Read the model definition and answer for the solid it produces. Units are mm, in the model's axes. A direction names the side the tool comes from. Coordinates: 2 decimals unless noted, no trailing zeros. Write each loop counter-clockwise with the first axis right and the second up, starting at its lowest first coordinate (ties: lowest second). Pieces come first, ordered by that corner, then holes.
(1) Which of the six approach directions +Z, -Z, +X, -X, +Y, -Y give full straight-line access (tool end or side, diameter ignored) to faces 4 (the flat face through (-49, -5.75, 4)), 5 (the cylindrical face through (46.38, 6.13, 5.05)), 6 (the flat face through (-49, 0, 5.4)), 7 (the flat face through (-49, 0, 5.6)), 8 (the flat face through (-17, 19.5, 4))?
(2) The part is cut by section D-D, the plane x = 31.6. Determine the outline of the cut face in (y, z).
(3) The part is cut by section A-A, the plane x = -48.85. Determine the outline of the cut face in (y, z) (3 decimals), and give its area (3 significant figures).
(4) Straight lines are drawn through the part: line 1 along Y through (x, z) = (46.1, 1.05); line 2 along Y through (x, z) = (5, 6); line 3 along Y through (x, z) = (-48.85, 0.85) (3 decimals). For each, find the intervals that lie inside material, in ascending order.
(5) Given pin 1 (4 mm diameter, centred on x = -48, y = 1.5, fed in from +Z); pin 2 (5.5 mm diameter, centred on x = 46.1, y = -19.5, fed in from +Z); pin 3 (0.7 mm diameter, centred on y = 1.5, z = 4.5, fed in from -X); pin 4 (1.5 mm diameter, centred on y = -18.5, z = 2.5, fed in from -X), each flat-ended and moving along its own axis, determine where each tip first touches the part or whether it passes through.
(6) The part is cut by section B-B, the plane y = -19.5. Determine the outline of the cut face in (x, z).
(7) The part is cut by section C-C, the plane y = 0. Determine the outline of the cut face in (x, z).
(8) Determine the mould class of faces 1 (the flat face through (-19, -14, 6.6)), 2 (the flat face through (-49, 0, 4.1)), 3 (the flat face through (-16, -14.5, 4)) for opening direction Y: pulls with the +Y half, pulls with the -Y half, needs draft (parallel to the pull), parting line crosses it, or undercut.
Autodesk Inventor part; units mm, degrees
ref_plane "YZ Plane" through (0, 0, 0) normal (1, 0, 0) x (0, 1, 0)
ref_plane "XZ Plane" through (0, 0, 0) normal (0, 1, 0) x (-1, 0, 0)
ref_plane "XY Plane" through (0, 0, 0) normal (0, 0, 1) x (1, 0, 0)
sketch "Sketch1" plane through (0, 0, 0) normal (0, 0, 1) x (1, 0, 0)
  line L0 (-52.6, 23) -> (52.6, 23)
  line L1 (52.6, 23) -> (52.6, -23)
  line L2 (52.6, -23) -> (-52.6, -23)
  line L3 (-52.6, -23) -> (-52.6, 23)
  point P0 (0, 0)
  point P1 (-52.6, 0)
  point P2 (0, 23)
  dimension "d0" = 105.2
  dimension "d2" = 46
extrude "Extrusion1" add sketch "Sketch1" along normal blind 1.6
sketch "Sketch2" plane through (0, 0, 1.6) normal (0, 0, 1) x (1, 0, 0)
  line L0 (-52.6, -23) -> (52.6, -23)
  line L1 (52.6, -23) -> (52.6, 23)
  line L2 (-45.1, 19.5) -> (12.4, 19.5)
  line L3 (12.4, 19.5) -> (12.4, -14.5)
  line L4 (12.4, -14.5) -> (-45.1, -14.5)
  line L5 (-45.1, -14.5) -> (-45.1, 19.5)
  circle A0 centre (31.6, 0) radius 16
  line L6 (31.6, 0) -> (31.6, -16)
  line L7 (31.6, 0) -> (31.6, 16)
  line L8 (52.6, 23) -> (-52.6, 23)
  line L9 (-52.6, 23) -> (-52.6, -23)
  point P0 (0, 0)
  dimension "d5" = 57.5
  dimension "d7" = 34
  dimension "d8" = 32
  dimension "d9" = 21
  dimension "d10" = 23
  dimension "d13" = 3.5
  dimension "d14" = 7.5
extrude "Extrusion2" add sketch "Sketch2" along normal blind 7 contours L2 L3 L4 L5 | A0 L6 L7 | L7 L6 A0
sketch "Sketch3" plane through (0, 0, 8.6) normal (0, 0, 1) x (1, 0, 0)
  line L0 (12.4, 19.5) -> (-45.1, 19.5)
  line L1 (-45.1, 19.5) -> (-45.1, -14.5)
  line L2 (-45.1, -14.5) -> (12.4, -14.5)
  line L3 (12.4, -14.5) -> (12.4, 19.5)
  point P0 (0, 0)
extrude "Extrusion3" cut sketch "Sketch3" against normal blind 2
sketch "Sketch4" plane through (0, 0, 6.6) normal (0, 0, 1) x (1, 0, 0)
  line L0 (-45.1, 19.5) -> (12.4, 19.5)
  line L1 (-45.1, -14.5) -> (-45.1, 19.5)
  line L2 (-42.5865, 18.0138) -> (9.8865, 18.0138)
  line L3 (9.8865, 18.0138) -> (9.8865, -13.0138)
  line L4 (9.8865, -13.0138) -> (-42.5865, -13.0138)
  line L5 (-42.5865, -13.0138) -> (-42.5865, 18.0138)
  line L6 (-45.1, -14.5) -> (-42.5865, -13.0138) construction
  point P0 (0, 0)
  point P1 (-45.1, 2.5)
  point P2 (-42.5865, 2.5)
  point P3 (-16.35, 18.0138)
  point P4 (-16.35, 19.5)
  dimension "d21" = 60.96
extrude "Extrusion4" cut sketch "Sketch4" against normal blind 1
sketch "Sketch5" plane through (0, 0, 1.6) normal (0, 0, 1) x (1, 0, 0)
  line L0 (-52.6, 23) -> (-52.6, -23)
  line L1 (-52.6, -5.75) -> (-45.1, -5.75)
  line L2 (-45.1, -5.75) -> (-45.1, 5.75)
  line L3 (-45.1, 5.75) -> (-52.6, 5.75)
  line L4 (-52.6, 5.75) -> (-52.6, -5.75)
  line L5 (-45.1, -14.5) -> (-45.1, 19.5)
  point P0 (0, 0)
  point P1 (-45.1, 0)
  point P2 (-52.6, 0)
  dimension "d24" = 11.5
extrude "Extrusion5" add sketch "Sketch5" along normal blind 4
sketch "Sketch6" plane through (-52.6, -23, 0) normal (-1, 0, 0) x (0, 0, 1)
  line L0 (1.6, 17.25) -> (5.6, 17.25)
  line L1 (5.6, 28.75) -> (5.6, 17.25)
  line L2 (1.6, 28.75) -> (5.6, 28.75)
  line L3 (1.6, 46) -> (1.6, 28.75)
  line L4 (4.1, 28.55) -> (5.4, 28.55)
  line L5 (5.4, 28.55) -> (5.4, 17.45)
  line L6 (5.4, 17.45) -> (4.1, 17.45)
  line L7 (4.1, 17.45) -> (4.1, 28.55)
  point P0 (0, 23)
  dimension "d28" = 2.5
  dimension "d29" = 0.2
  dimension "d30" = 0.2
  dimension "d31" = 0.2
extrude "Extrusion6" cut sketch "Sketch6" against normal up to surface (7.5 mm away)
sketch "Sketch7" plane through (0, 0, 1.6) normal (0, 0, 1) x (1, 0, 0)
  line L0 (52.6, -23) -> (52.6, 23)
  line L1 (-52.6, 23) -> (-52.6, 5.75)
  line L2 (-45.1, -14.5) -> (-45.1, -5.75)
  circle A0 centre (-48.85, -10.125) radius 1.75
  circle A1 centre (-48.85, 10.125) radius 1.75
  circle A2 centre (46.1, 19.5) radius 1.75
  circle A3 centre (46.1, -19.5) radius 1.75
  line L3 (-48.85, 10.125) -> (-48.85, -10.125) construction
  line L4 (46.1, 19.5) -> (46.1, -19.5) construction
  point P0 (0, 0)
  point P1 (52.6, 0)
  point P2 (-48.85, 0)
  point P3 (46.1, 0)
  point P4 (52.6, 0)
  point P5 (52.6, 0)
  dimension "d34" = 20.25
  dimension "d36" = 3.75
  dimension "d37" = 39
  dimension "d39" = 6.5
  dimension "d40" = 3.5
extrude "Extrusion7" cut sketch "Sketch7" against normal through all
properties part number "miniviki"
Computed:
1. face 4: +Z, -X, -Y
1. face 5: +Z
1. face 6: -X
1. face 7: +Z, -X, +Y, -Y
1. face 8: +Z, +X, -X, +Y
2. outline: (-23, 0) - (23, 0) - (23, 1.6) - (16, 1.6) - (16, 8.6) - (-16, 8.6) - (-16, 1.6) - (-23, 1.6) - close
3. outline: (-23, 0) - (-11.875, 0) - (-11.875, 1.6) - (-23, 1.6) - close; (-8.375, 0) - (8.375, 0) - (8.375, 1.6) - (5.75, 1.6) - (5.75, 5.6) - (-5.75, 5.6) - (-5.75, 1.6) - (-8.375, 1.6) - close; (11.875, 0) - (23, 0) - (23, 1.6) - (11.875, 1.6) - close; hole (-5.55, 4.1) - (5.55, 4.1) - (5.55, 5.4) - (-5.55, 5.4) - close
3. area: 94.0 mm2
4. line 1: y = -23 to -21.25, -17.75 to 17.75, 21.25 to 23
4. line 2: y = -14.5 to -13.01, 18.01 to 19.5
4. line 3: y = -23 to -11.875, -8.375 to 8.375, 11.875 to 23
5. pin 1: stops at z = 5.6
5. pin 2: stops at z = 1.6
5. pin 3: stops at x = -45.1
5. pin 4: passes through
6. outline: (-52.6, 0) - (44.35, 0) - (44.35, 1.6) - (-52.6, 1.6) - close; (47.85, 0) - (52.6, 0) - (52.6, 1.6) - (47.85, 1.6) - close
7. outline: (-52.6, 0) - (52.6, 0) - (52.6, 1.6) - (47.6, 1.6) - (47.6, 8.6) - (15.6, 8.6) - (15.6, 1.6) - (12.4, 1.6) - (12.4, 6.6) - (9.89, 6.6) - (9.89, 5.6) - (-42.59, 5.6) - (-42.59, 6.6) - (-45.1, 6.6) - (-45.1, 5.6) - (-52.6, 5.6) - (-52.6, 5.4) - (-45.1, 5.4) - (-45.1, 4.1) - (-52.6, 4.1) - close
8. face 1: needs draft
8. face 2: undercut
8. face 3: pulls with the -Y half
